The model under review builds one solid part; all positions refer to its coordinate system, in mm. A direction names the side the tool comes from. Round coordinates to 2 decimals unless told otherwise and drop trailing zeros. Loops run counter-clockwise (first coordinate to the right, second up) from the corner with the lowest first, then second, coordinate; pieces in that order, holes last. Notation, with made-up numbers: M 48.25,5.5 L 59.25,5.5 A20 cw 59.25,25.5 Z; hole C 75,17.25 d1. An arc over 180 degrees is marked long. Return JSON: item names as keys, results as strings. Group by question number.
Q1. Consider section A-A (y = -36.5). State the section outline as (x, z) points (3 decimals).
Q2. Consider section C-C (y = 60). State the section outline as (x, z) points, and give its area (3 significant figures).
Q3. Clearance check with flat-ended pins moving along their axes: pin 1 Ø0.6 at (x, z) = (-79, 1) entering from +Y; pin 2 Ø1 at (y, z) = (75.5, 0) entering from +X; pin 3 Ø1 at (x, z) = (75.5, 1) entering from +Y. State where each tip first meets the part, or that it passes through.
Q4. Consider section D-D (z = 1.4). Count the separate pieces of the cut face and the enclosed holes in it, and give its area (3 significant figures).
Q5. For faces 4 (the face through (46.984, 88.601, 0.986)), 5 (the face through (-2, -19, 0)), list the 3-axis set-ups (+Z, -Z, +X, -X, +Y, -Y) from which the entire face can be reached by the end or side of a thin tool; tool diameter is ignored.
Q6. Draft analysis for pull direction Y (two halves, no side actions). For faces 1 (the face through (-63.66, 74.39, 0.99)), 2 (the face through (60.141, 88.236, 0.986)), 3 (the face through (-2, -19, 2)), state which applies: pulls with the +Y half, pulls with the -Y half, needs draft (parallel to the pull), parting line crosses it, or undercut.
Q7. To check wall thickness, follow line 1 along Y through (x, z) = (-13, 1.7); line 2 along Y through (x, z) = (15.5, 0.3); line 3 along X through (y, z) = (-38, 1.9) (3 decimals). State the ranges of each line that lie inside material, in increasing order.
Q8. Consider section B-B (x = 18.5). State the section outline as (y, z) points, and give its area (3 significant figures).
Autodesk Inventor part; units mm, degrees
ref_plane "YZ Plane" through (0, 0, 0) normal (1, 0, 0) x (0, 1, 0)
ref_plane "XZ Plane" through (0, 0, 0) normal (0, 1, 0) x (-1, 0, 0)
ref_plane "XY Plane" through (0, 0, 0) normal (0, 0, 1) x (1, 0, 0)
sketch "Sketch1" plane through (0, 0, 0) normal (0, 0, 1) x (1, 0, 0)
  line L0 (-77.4547, 22.5062) -> (-79.4547, 22.5062)
  line L1 (-88.4548, -106.3305) -> (-88.4548, 62.3216)
  line L2 (-77.4547, -10.4938) -> (-79.4547, -10.4938)
  line L3 (-77.4547, 4.5062) -> (-77.4547, -10.4938)
  line L4 (-79.4547, 4.5062) -> (-77.4547, 4.5062)
  line L5 (-79.4547, -10.4938) -> (-79.4547, 4.5062)
  line L6 (-77.4547, 37.5062) -> (-77.4547, 22.5062)
  line L7 (-79.4547, 37.5062) -> (-77.4547, 37.5062)
  line L8 (-79.4547, 22.5062) -> (-79.4547, 37.5062)
  line L9 (-77.4547, -42.4938) -> (-79.4547, -42.4938)
  line L10 (-77.4547, -27.4938) -> (-77.4547, -42.4938)
  line L11 (-79.4547, -42.4938) -> (-79.4547, -27.4938)
  line L12 (-79.4547, -27.4938) -> (-77.4547, -27.4938)
  line L13 (-58.1998, -33.3656) -> (-45.1998, -33.3656)
  line L14 (-45.1998, -33.3656) -> (-45.1998, -12.3656)
  line L15 (-58.1998, -12.3656) -> (-58.1998, -33.3656)
  line L16 (-45.1998, -12.3656) -> (-58.1998, -12.3656)
  line L17 (-79.4548, -60.4938) -> (-77.4548, -60.4938)
  line L18 (-77.4548, -60.4938) -> (-77.4548, -75.4938)
  line L19 (-79.4548, -75.4938) -> (-79.4548, -60.4938)
  line L20 (-77.4548, -75.4938) -> (-79.4548, -75.4938)
  circle A0 centre (-70.4548, -88.3305) radius 1.5
  line L21 (-57.6182, -95.3305) -> (-42.6182, -95.3305)
  line L22 (-42.6182, -95.3305) -> (-42.6182, -97.3305)
  line L23 (-42.6182, -97.3305) -> (-57.6182, -97.3305)
  line L24 (-57.6182, -97.3305) -> (-57.6182, -95.3305)
  line L25 (-65.7269, 69.4932) -> (-67.1411, 70.9074)
  line L26 (-60.0701, 77.9785) -> (-58.6558, 76.5643)
  line L27 (-58.6558, 76.5643) -> (-65.7269, 69.4932)
  line L28 (-67.1411, 70.9074) -> (-60.0701, 77.9785)
  line L29 (-45.9277, 92.1205) -> (-44.5135, 90.7062)
  line L30 (-44.5135, 90.7062) -> (-51.5846, 83.6352)
  line L31 (-52.9988, 85.0494) -> (-45.9277, 92.1205)
  line L32 (-88.4548, 62.3216) -> (-37.342, 113.4344)
  line L33 (-51.5846, 83.6352) -> (-52.9988, 85.0494)
  line L34 (-37.0998, 52.6344) -> (-37.0998, 78.4344)
  line L35 (-16.1999, 102.4344) -> (-16.1999, 104.4344)
  line L36 (-6.1999, 102.4344) -> (-16.1999, 102.4344)
  line L37 (-16.1999, 104.4344) -> (-6.1999, 104.4344)
  line L38 (-6.1999, 104.4344) -> (-6.1999, 102.4344)
  line L39 (3.8002, 102.4342) -> (3.8002, 104.4342)
  line L40 (13.8002, 102.4342) -> (3.8002, 102.4342)
  line L41 (13.8002, 104.4342) -> (13.8002, 102.4342)
  line L42 (3.8002, 104.4342) -> (13.8002, 104.4342)
  line L43 (-37.0998, 78.4344) -> (34.7002, 78.4344)
  line L44 (-37.342, 113.4344) -> (34.9424, 113.4344)
  line L45 (34.7002, 52.6344) -> (-37.0998, 52.6344)
  line L46 (34.7002, 78.4344) -> (34.7002, 52.6344)
  line L47 (22.3818, -95.3307) -> (22.3818, -97.3307)
  line L48 (40.3818, -97.3307) -> (40.3818, -95.3307)
  line L49 (55.3818, -95.3307) -> (55.3818, -97.3307)
  line L50 (55.3818, -97.3307) -> (40.3818, -97.3307)
  line L51 (40.3818, -95.3307) -> (55.3818, -95.3307)
  line L52 (7.3818, -95.3307) -> (22.3818, -95.3307)
  line L53 (22.3818, -97.3307) -> (7.3818, -97.3307)
  line L54 (7.3818, -97.3307) -> (7.3818, -95.3307)
  line L55 (86.0552, -106.3305) -> (-88.4548, -106.3305)
  line L56 (-9.6182, -95.3307) -> (-9.6182, -97.3307)
  line L57 (-24.6182, -95.3307) -> (-9.6182, -95.3307)
  line L58 (-24.6182, -97.3307) -> (-24.6182, -95.3307)
  line L59 (-9.6182, -97.3307) -> (-24.6182, -97.3307)
  line L60 (86.0552, 62.3216) -> (86.0552, -106.3305)
  circle A1 centre (68.0552, -88.3305) radius 1.5
  line L61 (75.0552, -75.4938) -> (77.0552, -75.4938)
  line L62 (77.0552, -60.4938) -> (75.0552, -60.4938)
  line L63 (77.0552, -75.4938) -> (77.0552, -60.4938)
  line L64 (75.055, -42.4938) -> (77.055, -42.4938)
  line L65 (75.055, -27.4938) -> (75.055, -42.4938)
  line L66 (77.055, -42.4938) -> (77.055, -27.4938)
  line L67 (75.0552, -60.4938) -> (75.0552, -75.4938)
  line L68 (42.8002, -12.3656) -> (55.8002, -12.3656)
  line L69 (77.055, 4.5062) -> (75.055, 4.5062)
  line L70 (75.055, 4.5062) -> (75.055, -10.4938)
  line L71 (77.055, -10.4938) -> (77.055, 4.5062)
  line L72 (42.8002, -33.3656) -> (42.8002, -12.3656)
  line L73 (75.055, -10.4938) -> (77.055, -10.4938)
  line L74 (55.8002, -12.3656) -> (55.8002, -33.3656)
  line L75 (55.8002, -33.3656) -> (42.8002, -33.3656)
  line L76 (77.055, -27.4938) -> (75.055, -27.4938)
  line L77 (77.055, 37.5062) -> (75.055, 37.5062)
  line L78 (75.055, 22.5062) -> (77.055, 22.5062)
  line L79 (77.055, 22.5062) -> (77.055, 37.5062)
  line L80 (75.055, 37.5062) -> (75.055, 22.5062)
  circle A2 centre (48.8002, 27.6344) radius 8
  circle A3 centre (68.0552, 54.8658) radius 1.5
  line L81 (64.6739, 70.8372) -> (63.2567, 69.426)
  line L82 (63.2567, 69.426) -> (56.2003, 76.5117)
  line L83 (56.2003, 76.5117) -> (57.6175, 77.9229)
  line L84 (57.6175, 77.9229) -> (64.6739, 70.8372)
  line L85 (50.5611, 85.0087) -> (49.1439, 83.5974)
  line L86 (49.1439, 83.5974) -> (42.0875, 90.6831)
  line L87 (42.0875, 90.6831) -> (43.5047, 92.0944)
  line L88 (43.5047, 92.0944) -> (50.5611, 85.0087)
  line L89 (34.9424, 113.4344) -> (86.0552, 62.3216)
  circle A4 centre (-70.4548, 54.8658) radius 1.5
  circle A5 centre (-51.1998, 27.6344) radius 8
  circle A6 centre (-1.1998, 32.6344) radius 4.85
  point P0 (0, 0)
  dimension "d44" = 10
  dimension "d45" = 2
  dimension "d46" = 10
  dimension "d47" = 2
  dimension "d48" = 10
  dimension "d49" = 2
  dimension "d50" = 10
  dimension "d51" = 2
  dimension "d52" = 10
  dimension "d53" = 10
  dimension "d54" = 2
  dimension "d55" = 10
  dimension "d56" = 2
  dimension "d57" = 10
  dimension "d58" = 15
  dimension "d59" = 2
  dimension "d60" = 15
  dimension "d61" = 18
  dimension "d62" = 15
  dimension "d63" = 17
  dimension "d64" = 2
  dimension "d65" = 15
  dimension "d66" = 15
  dimension "d67" = 18
  dimension "d68" = 15
  dimension "d69" = 17
  dimension "d70" = 15
  dimension "d71" = 18
  dimension "d72" = 15
  dimension "d73" = 18
  dimension "d74" = 219.7649
  dimension "d75" = 174.51
  dimension "d76" = 3
  dimension "d77" = 3
  dimension "d78" = 71.8
  dimension "d79" = 25.8
  dimension "d80" = 35
  dimension "d81" = 16
  dimension "d82" = 25
  dimension "d83" = 13
  dimension "d84" = 21
  dimension "d85" = 40
  dimension "d86" = 9.7
  dimension "d87" = 20
extrude "Extrusion1" add sketch "Sketch1" along normal blind 2 contours L1 L32 L44 L89 L60 L55 | A0 | A1 | A3 | A4
sketch "Sketch2" plane through (0, 0, 2) normal (0, 0, 1) x (1, 0, 0)
  line L0 (-77.4547, -10.4938) -> (-79.4547, -10.4938)
  line L1 (-45.1998, -12.3656) -> (-58.1998, -12.3656)
  line L2 (-79.4547, 4.5062) -> (-77.4547, 4.5062)
  line L3 (-77.4547, 4.5062) -> (-77.4547, -10.4938)
  line L4 (-79.4547, -10.4938) -> (-79.4547, 4.5062)
  line L5 (-77.4547, 22.5062) -> (-79.4547, 22.5062)
  line L6 (-24.6182, -97.3307) -> (-24.6182, -95.3307)
  line L7 (-9.6182, -95.3307) -> (-9.6182, -97.3307)
  line L8 (-24.6182, -95.3307) -> (-9.6182, -95.3307)
  line L9 (-9.6182, -97.3307) -> (-24.6182, -97.3307)
  line L10 (-45.9277, 92.1205) -> (-44.5135, 90.7062)
  line L11 (-44.5135, 90.7062) -> (-51.5846, 83.6352)
  line L12 (-52.9988, 85.0494) -> (-45.9277, 92.1205)
  line L13 (-51.5846, 83.6352) -> (-52.9988, 85.0494)
  line L14 (-60.0701, 77.9785) -> (-58.6558, 76.5643)
  line L15 (-58.6558, 76.5643) -> (-65.7269, 69.4932)
  line L16 (-67.1411, 70.9074) -> (-60.0701, 77.9785)
  line L17 (-65.7269, 69.4932) -> (-67.1411, 70.9074)
  line L18 (-88.4548, 62.3216) -> (-37.342, 113.4344)
  line L19 (-88.4548, -106.3305) -> (-88.4548, 62.3216)
  line L20 (-58.1998, -12.3656) -> (-58.1998, -33.3656)
  line L21 (-45.1998, -33.3656) -> (-45.1998, -12.3656)
  line L22 (-79.4547, -27.4938) -> (-77.4547, -27.4938)
  line L23 (-58.1998, -33.3656) -> (-45.1998, -33.3656)
  line L24 (-79.4547, -42.4938) -> (-79.4547, -27.4938)
  line L25 (-77.4547, -27.4938) -> (-77.4547, -42.4938)
  line L26 (-77.4547, -42.4938) -> (-79.4547, -42.4938)
  line L27 (7.3818, -97.3307) -> (7.3818, -95.3307)
  line L28 (7.3818, -95.3307) -> (22.3818, -95.3307)
  line L29 (22.3818, -97.3307) -> (7.3818, -97.3307)
  line L30 (40.3818, -97.3307) -> (40.3818, -95.3307)
  line L31 (55.3818, -95.3307) -> (55.3818, -97.3307)
  line L32 (22.3818, -95.3307) -> (22.3818, -97.3307)
  line L33 (-16.1999, 102.4344) -> (-16.1999, 104.4344)
  line L34 (-6.1999, 102.4344) -> (-16.1999, 102.4344)
  line L35 (-16.1999, 104.4344) -> (-6.1999, 104.4344)
  line L36 (-6.1999, 104.4344) -> (-6.1999, 102.4344)
  line L37 (3.8002, 102.4342) -> (3.8002, 104.4342)
  line L38 (13.8002, 102.4342) -> (3.8002, 102.4342)
  line L39 (13.8002, 104.4342) -> (13.8002, 102.4342)
  line L40 (3.8002, 104.4342) -> (13.8002, 104.4342)
  circle A0 centre (-1.1998, 32.6344) radius 4.85
  line L41 (42.0875, 90.6831) -> (43.5047, 92.0944)
  line L42 (-37.0998, 52.6344) -> (-37.0998, 78.4344)
  line L43 (34.7002, 78.4344) -> (34.7002, 52.6344)
  line L44 (34.7002, 52.6344) -> (-37.0998, 52.6344)
  line L45 (-37.0998, 78.4344) -> (34.7002, 78.4344)
  line L46 (-37.342, 113.4344) -> (34.9424, 113.4344)
  line L47 (86.0552, -106.3305) -> (-88.4548, -106.3305)
  line L48 (-42.6182, -95.3305) -> (-42.6182, -97.3305)
  line L49 (-42.6182, -97.3305) -> (-57.6182, -97.3305)
  line L50 (-57.6182, -95.3305) -> (-42.6182, -95.3305)
  line L51 (-57.6182, -97.3305) -> (-57.6182, -95.3305)
  circle A1 centre (-70.4548, -88.3305) radius 1.5
  line L52 (-77.4548, -60.4938) -> (-77.4548, -75.4938)
  line L53 (-79.4548, -60.4938) -> (-77.4548, -60.4938)
  line L54 (-79.4548, -75.4938) -> (-79.4548, -60.4938)
  line L55 (-77.4548, -75.4938) -> (-79.4548, -75.4938)
  line L56 (55.3818, -97.3307) -> (40.3818, -97.3307)
  line L57 (40.3818, -95.3307) -> (55.3818, -95.3307)
  circle A2 centre (68.0552, -88.3305) radius 1.5
  line L58 (75.0552, -60.4938) -> (75.0552, -75.4938)
  line L59 (77.0552, -60.4938) -> (75.0552, -60.4938)
  line L60 (77.0552, -75.4938) -> (77.0552, -60.4938)
  line L61 (86.0552, 62.3216) -> (86.0552, -106.3305)
  line L62 (75.055, -42.4938) -> (77.055, -42.4938)
  line L63 (75.0552, -75.4938) -> (77.0552, -75.4938)
  line L64 (75.055, -27.4938) -> (75.055, -42.4938)
  line L65 (77.055, -42.4938) -> (77.055, -27.4938)
  line L66 (77.055, -27.4938) -> (75.055, -27.4938)
  line L67 (55.8002, -33.3656) -> (42.8002, -33.3656)
  line L68 (75.055, -10.4938) -> (77.055, -10.4938)
  line L69 (42.8002, -12.3656) -> (55.8002, -12.3656)
  line L70 (42.8002, -33.3656) -> (42.8002, -12.3656)
  line L71 (77.055, -10.4938) -> (77.055, 4.5062)
  line L72 (77.055, 4.5062) -> (75.055, 4.5062)
  line L73 (75.055, 4.5062) -> (75.055, -10.4938)
  line L74 (55.8002, -12.3656) -> (55.8002, -33.3656)
  line L75 (64.6739, 70.8372) -> (63.2567, 69.426)
  line L76 (63.2567, 69.426) -> (56.2003, 76.5117)
  line L77 (56.2003, 76.5117) -> (57.6175, 77.9229)
  line L78 (57.6175, 77.9229) -> (64.6739, 70.8372)
  line L79 (50.5611, 85.0087) -> (49.1439, 83.5974)
  line L80 (49.1439, 83.5974) -> (42.0875, 90.6831)
  line L81 (43.5047, 92.0944) -> (50.5611, 85.0087)
  line L82 (34.9424, 113.4344) -> (86.0552, 62.3216)
  line L83 (75.055, 22.5062) -> (77.055, 22.5062)
  line L84 (77.055, 37.5062) -> (75.055, 37.5062)
  line L85 (77.055, 22.5062) -> (77.055, 37.5062)
  line L86 (75.055, 37.5062) -> (75.055, 22.5062)
  circle A3 centre (68.0552, 54.8658) radius 1.5
  circle A4 centre (48.8002, 27.6344) radius 8
  circle A5 centre (-51.1998, 27.6344) radius 8
  line L87 (-77.4547, 37.5062) -> (-77.4547, 22.5062)
  line L88 (-79.4547, 22.5062) -> (-79.4547, 37.5062)
  line L89 (-79.4547, 37.5062) -> (-77.4547, 37.5062)
  circle A6 centre (-70.4548, 54.8658) radius 1.5
  point P0 (0, 0)
  point P1 (0, 0)
  dimension "d90" = 10
  dimension "d91" = 2
  dimension "d92" = 10
  dimension "d93" = 2
  dimension "d94" = 10
  dimension "d95" = 2
  dimension "d96" = 10
  dimension "d97" = 2
  dimension "d98" = 10
  dimension "d99" = 10
  dimension "d100" = 2
  dimension "d101" = 10
  dimension "d102" = 2
  dimension "d103" = 10
  dimension "d104" = 15
  dimension "d105" = 2
  dimension "d106" = 15
  dimension "d107" = 18
  dimension "d108" = 15
  dimension "d109" = 17
  dimension "d110" = 2
  dimension "d111" = 15
  dimension "d112" = 15
  dimension "d113" = 18
  dimension "d114" = 15
  dimension "d115" = 17
  dimension "d116" = 15
  dimension "d117" = 18
  dimension "d118" = 15
  dimension "d119" = 18
  dimension "d120" = 219.7649
  dimension "d121" = 174.51
  dimension "d122" = 3
  dimension "d123" = 3
  dimension "d124" = 71.8
  dimension "d125" = 25.8
  dimension "d126" = 35
  dimension "d127" = 16
  dimension "d128" = 25
  dimension "d129" = 13
  dimension "d130" = 21
  dimension "d131" = 40
  dimension "d132" = 9.7
  dimension "d133" = 20
hole "Hole1" at (-70.4548, 54.8658, 2) at (68.0552, 54.8658, 2) at (68.0552, -88.3305, 2) at (-70.4548, -88.3305, 2) direction (0, 0, -1) diameter 3 end through all
properties part number "tutup kepala"
Values:
{
 "1": {"outline": "M -88.455,0 L -79.455,0 L -79.455,2 L -88.455,2 Z; M -77.455,0 L 75.055,0 L 75.055,2 L -77.455,2 Z; M 77.055,0 L 86.055,0 L 86.055,2 L 77.055,2 Z"},
 "2": {"outline": "M -88.45,0 L -37.1,0 L -37.1,2 L -88.45,2 Z; M 34.7,0 L 86.06,0 L 86.06,2 L 34.7,2 Z", "area": "205 mm2"},
 "3": {"pin 1": "stops at y = 72.08", "pin 2": "stops at x = 73.38", "pin 3": "stops at y = 73.38"},
 "4": {"separate pieces": "1", "enclosed holes": "28", "area": "32,400 mm2"},
 "5": {"face 4": "+Z, -Z", "face 5": "-Z, +X, -X, +Y, -Y"},
 "6": {"face 1": "undercut", "face 2": "pulls with the +Y half", "face 3": "needs draft"},
 "7": {"line 1": "y = -106.33 to -97.33, -95.33 to 52.63, 78.43 to 102.43, 104.43 to 113.43", "line 2": "y = -106.33 to -97.33, -95.33 to 52.63, 78.43 to 113.43", "line 3": "x = -88.455 to -79.455, -77.455 to 75.055, 77.055 to 86.055"},
 "8": {"outline": "M -106.33,0 L -97.33,0 L -97.33,2 L -106.33,2 Z; M -95.33,0 L 52.63,0 L 52.63,2 L -95.33,2 Z; M 78.43,0 L 113.43,0 L 113.43,2 L 78.43,2 Z", "area": "384 mm2"}
}
